Work out the finished part from the listing and answer in its coordinate system (mm). A direction names the side the tool comes from. Round coordinates to 2 decimals unless told otherwise and drop trailing zeros. Order: outer loops, then holes, each group sorted by start corner. A loop starts at its lowest first (then second) coordinate and runs counter-clockwise, first axis right, second up. Notation, with made-up numbers: (70.25, -28.75) -> (85.25, -28.75) arc R25 cw to (85.25, 1.25) -> close; hole circle Ø1 at (45, -27.5). An arc over 180 degrees is marked (long way). Use one line per item in the form item = value.
```python
from build123d import *

# Parameters (mm, degrees)
F0_W      = 20
F0_H      = 20
F1_DEPTH  = 1.5
F2_W      = 3
F2_H      = 14
F3_DEPTH  = 1.5
F4_W      = 1.5
F4_H      = 14
F5_DEPTH  = 1.5
F6_DEPTH  = 6
F7_W      = 17
F7_H      = 17
F8_DEPTH  = 1.5
F9_W      = 2.5
F9_H      = 1
F10_DEPTH = 20
F11_R     = 0.99999
F12_R     = 0.5
F13_SIZE  = 0.5


# Not quite as in the source:
# - a fillet or chamfer is up to 0.001 mm smaller than in the source, because OpenCascade refuses the exact size


with BuildPart() as f1:
    # F0 (on Top) → F1 (new body)
    with BuildSketch(Plane.XY):
        Rectangle(F0_W, F0_H)
    extrude(amount=F1_DEPTH)

    # F6 (add): a face of the model
    f6_faces = [f1.faces().sort_by_distance(p)[0] for p in [
        (0, 0, 1.5),
    ]]


with BuildPart() as f3:
    # F2 (on face) → F3 (new body)
    with BuildSketch(Plane.XY.offset(1.5)):
        with Locations((-11.5, 0)):
            Rectangle(F2_W, F2_H)
    extrude(amount=F3_DEPTH)

    # F4 (on face) → F5 (join)
    with BuildSketch(Plane.XY.offset(3)):
        with Locations((-12.25, 0)):
            Rectangle(F4_W, F4_H)
    extrude(amount=F5_DEPTH)


with BuildPart() as f1_1:
    add(f1.part)

    add(f3.part)  # F6 merges F3
    extrude(f6_faces, amount=F6_DEPTH)

    # F7 (on face) → F8 (cut)
    with BuildSketch(Plane.XY.offset(7.5)):
        Rectangle(F7_W, F7_H)
    extrude(amount=-F8_DEPTH, mode=Mode.SUBTRACT)

    # F9 (on face) → F10 (cut, through all)
    with BuildSketch(Plane.XZ.offset(10)):
        Polygon((6.5, 1), (10, 1), (10, 4), (9, 4), (6.5, 4), align=None)
        with Locations((7.75, 4.5)):
            Rectangle(F9_W, F9_H)
    extrude(amount=-F10_DEPTH, mode=Mode.SUBTRACT)

    # F11 (radius 1 in the source; OpenCascade refuses exactly that, so slightly less here)
    f11_edges = [f1_1.edges().sort_by_distance(p)[0] for p in [
        (6.5, 0, 5),
        (9, 0, 5),
    ]]
    fillet(f11_edges, radius=F11_R)

    # F12
    f12_edges = [f1_1.edges().sort_by_distance(p)[0] for p in [
        (-10, 0, 3),
    ]]
    fillet(f12_edges, radius=F12_R)

    # F13
    f13_edges = [f1_1.edges().sort_by_distance(p)[0] for p in [
        (0, -10, 0),
        (10, 0, 0),
        (0, 10, 0),
        (-10, 0, 0),
    ]]
    chamfer(f13_edges, length=F13_SIZE)


solid = f1_1.part
```
Item 1: For faces 5 (the flat face through (-12, 0, 1.5)), 6 (the cylindrical face through (6.785, 0.14, 4.699)), 7 (the flat face through (8.5, 0, 7)), determine the directions among +Z, -Z, +X, -X, +Y, -Y from which every point of the face is accessible in a straight line to the end or side of a thin tool.
Findings:
face_5 = -Z, -X, +Y, -Y
face_6 = +Y, -Y
face_7 = +Z
Item 2: Consider line 1 along Y through (x, z) = (3.75, 6.75); line 2 along X through (y, z) = (-8, 1.75). Determine where each line is inside the solid, lowest interval first.
Findings:
line_1 = -10 to -8.5, 8.5 to 10
line_2 = -10 to 6.5
Item 3: The part is cut by section A-A, the plane z = 7. Give the vertices of the cut face in (x, y).
Findings:
outline = (-10, -10) -> (10, -10) -> (10, 10) -> (-10, 10) -> close; hole (-8.5, -8.5) -> (8.5, -8.5) -> (8.5, 8.5) -> (-8.5, 8.5) -> close
Item 4: Flat-ended cylindrical pins translate along their axes: P1, Ø2.5, axis at x = -12, z = 2.5, coming from the -Y side; P2, Ø2.5, axis at x = -11, y = -2, coming from the -Z side; P3, Ø1.2, axis at x = -12.5, y = 0, coming from the +Z side; P4, Ø2.5, axis at y = 1.5, z = 3, coming from the +X side. Find the tip coordinate at first contact, or state that the pin passes through.
Findings:
P1 = -7
P2 = 0.25
P3 = 4.5
P4 = 10
Item 5: The part is cut by section B-B, the plane x = -4.25. Give the vertices of the cut face in (y, z), and give its area (3 significant figures).
Findings:
outline = (-10, 0.5) -> (-9.5, 0) -> (9.5, 0) -> (10, 0.5) -> (10, 7.5) -> (8.5, 7.5) -> (8.5, 6) -> (-8.5, 6) -> (-8.5, 7.5) -> (-10, 7.5) -> close
area = 124 mm^2
Item 6: The part is cut by section D-D, the plane z = 2.5. Give the vertices of the cut face in (x, y).
Findings:
outline = (-13, -7) -> (-10, -7) -> (-10, -10) -> (6.5, -10) -> (6.5, 10) -> (-10, 10) -> (-10, 7) -> (-13, 7) -> close
Item 7: Determine the mould class of faces 1 (the flat face through (8, 0, 1)), 2 (the flat face through (9.5, -0.1, 4)), 3 (the flat face through (-12, -7, 3)), 4 (the flat face through (0, 0, 6)) for opening direction Z: released by +Z, released by -Z, zero draft, split by the parting line, or undercut.
Findings:
face_1 = undercut
face_2 = undercut
face_3 = zero draft
face_4 = released by +Z
